Could you check a few things on this model? Use its own coordinates, in mm. Face numbers are marked on the shaded views. A direction names the side the tool comes from. Coordinates: 2 decimals unless noted, no trailing zeros. Order: outer loops, then holes, each group sorted by start corner. A loop starts at its lowest first (then second) coordinate and runs counter-clockwise, first axis right, second up. Notation, with made-up numbers: M -5,-30 L 46,-30 A19 ccw 46,-23 Z; hole C 86,27 d3. An arc over 180 degrees is marked long. One line per question, with ' | ' between items. Start each with the question number.
from build123d import *

# Parameters (mm, degrees)
ESBO_O1_R                = 1.6
RESSALTO_EXTRUS_O1_DEPTH = 20
ESBO_O2_W                = 10
ESBO_O2_H                = 36.212539342
CORTE_EXTRUS_O1_DEPTH    = 17
CHANFRO1_SIZE            = 10
ESBO_O3_R                = 1.5
CORTE_EXTRUS_O2_DEPTH    = 7


with BuildPart() as part:
    # Esboço1 → Ressalto-extrusão1 (new body)
    with BuildSketch(Plane.XY):
        with BuildLine():
            Line((5, 12.5), (5, 6))
            Line((5, 6), (17, 6))
            Line((17, 6), (17, -4))
            Line((17, -4), (5, -4))
            Line((5, -4), (5, -12.5))
            ThreePointArc((5, -12.5), (0, -17.5), (-5, -12.5))
            Line((-5, -12.5), (-5, 12.5))
            ThreePointArc((-5, 12.5), (0, 17.5), (5, 12.5))
        make_face()
        with Locations((0, -12.5)):
            Circle(ESBO_O1_R, mode=Mode.SUBTRACT)
        with Locations((0, 12.5)):
            Circle(ESBO_O1_R, mode=Mode.SUBTRACT)
    extrude(amount=RESSALTO_EXTRUS_O1_DEPTH)

    # Esboço2 → Corte-extrusão1 (cut)
    with BuildSketch(Plane.XY.offset(20)):
        Rectangle(ESBO_O2_W, ESBO_O2_H)
    extrude(amount=-CORTE_EXTRUS_O1_DEPTH, mode=Mode.SUBTRACT)

    # Chanfro1
    chanfro1_edges = [part.edges().sort_by_distance(p)[0] for p in [
        (5, 1, 3),
    ]]
    chamfer(chanfro1_edges, length=CHANFRO1_SIZE - 0.0001)  # a hair under: the kernel refuses the full size

    # Esboço3 → Corte-extrusão2 (cut)
    # profile 1 of 2: a face of its own
    with BuildSketch(Plane(origin=(17, 0, 0), x_dir=(0, 0, -1), z_dir=(1, 0, 0))):
        with BuildLine():
            Line((0, 4.8), (-7.081235465, 4.8))
            ThreePointArc((-7.081235465, 4.8), (-9.523984558, 0.949792684), (-5, 0.379982867))
            Line((-5, 0.379982867), (-3, 2.8))
            Line((-3, 2.8), (0, 2.8))
            Line((0, 2.8), (0, 4.8))
        make_face()
        with Locations((-7.081235465, 2.1)):
            Circle(ESBO_O3_R, mode=Mode.SUBTRACT)
    # profile 2 of 2: a face of its own
    with BuildSketch(Plane(origin=(17, 0, 0), x_dir=(0, 0, -1), z_dir=(1, 0, 0))):
        with BuildLine():
            Line((-20, 4.8), (-20, 2.8))
            Line((-20, 2.8), (-17, 2.8))
            Line((-17, 2.8), (-15, 0.379982867))
            ThreePointArc((-15, 0.379982867), (-10.476015442, 0.949792684), (-12.918764535, 4.8))
            Line((-12.918764535, 4.8), (-20, 4.8))
        make_face()
        with Locations(Location((-12.918764535, 2.1, 0), (0, 0, 180))):
            Circle(ESBO_O3_R, mode=Mode.SUBTRACT)
    extrude(amount=-CORTE_EXTRUS_O2_DEPTH, mode=Mode.SUBTRACT)


solid = part.part
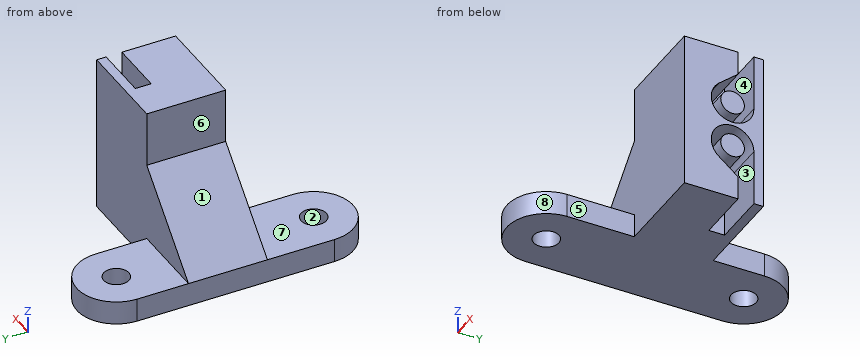
(1) Imagine slicing it at B-B, the plane z = 1.75. Write out the boundary of the cut face in (x, y), plus the area to 3 significant figures.
(2) Imagine slicing it at A-A, the plane x = 15.5. Write out the boundary of the cut face in (y, z), plus the area to 3 significant figures.
(3) For P1, Ø3.5, axis at y = 1.5, z = 15, coming from the -X side; P2, Ø5, axis at x = 1, y = -2.5, coming from the +Z side; P3, Ø4, axis at x = -1, y = 4.5, coming from the +Z side; P4, Ø1.9, axis at x = 0, y = -12.5, coming from the +Z side, each with a flat end and sliding along its axis, tell me the tip position at first contact or that it passes through.
(4) If I drill on line 1 along X through (y, z) = (12.5, 2.25); line 2 along Y through (x, z) = (11.25, 5.75); line 3 along Y through (x, z) = (7.75, 12), over which ranges is the centre line in solid material (lowest first)? Write a range as from..to.
(5) We'd pull the mould along X, two halves only. Please class the marked faces 1, 2 and 3: +X half, -X half, draft (parallel to the pull), parting line (faces both ways), or undercut.
(6) Imagine slicing it at C-C, the plane z = 18.5. Write out the boundary of the cut face in (x, y), plus the area to 3 significant figures.
(7) On a 3-axis mill with a long thin cutter (end or side, diameter ignored), from which of +Z, -Z, +X, -X, +Y, -Y can I reach the whole of each face in a straight line? I mean the marked faces 4, 5, 6, 7 and 8. Say none if no direction works.
Answers:
1) outline: M -5,-12.5 A5 ccw 5,-12.5 L 5,-4 L 17,-4 L 17,2.8 L 10,2.8 L 10,4.8 L 17,4.8 L 17,6 L 5,6 L 5,12.5 A5 ccw -5,12.5 Z; hole C 0,-12.5 d3.2; hole C 0,12.5 d3.2 | area: 418 mm²
2) outline: M -4,0 L 2.8,0 L 2.8,3 L 0.38,5 A2.7 cw long 4.8,7.08 L 4.8,0 L 6,0 L 6,20 L 4.8,20 L 4.8,12.92 A2.7 cw long 0.38,15 L 2.8,17 L 2.8,20 L -4,20 Z; C 2.1,7.08 d3; C 2.1,12.92 d3 | area: 145 mm²
3) P1: x = 5 | P2: z = 11.5 | P3: z = 9 | P4: through
4) line 1: -5..-1.6, 1.6..5 | line 2: -4..-0.25, 1.41..2.79, 4.8..6 | line 3: -4..6
5) face 1: -X half | face 2: undercut | face 3: draft
6) outline: M 5,-4 L 17,-4 L 17,2.8 L 10,2.8 L 10,4.8 L 17,4.8 L 17,6 L 5,6 Z | area: 106 mm²
7) face 4: +Z, +X | face 5: +Z, -Z, +X, -Y | face 6: +Z, -X, +Y, -Y | face 7: +Z, +X, -X | face 8: +Z, -Z, -Y
